Can you work these out from the model? Positions are in its coordinate system, mm. A direction names the side the tool comes from. Round coordinates to 2 decimals unless told otherwise and drop trailing zeros. Order: outer loops, then holes, each group sorted by start corner. A loop starts at its lowest first (then second) coordinate and runs counter-clockwise, first axis right, second up. Notation, with made-up numbers: M 25.5,56 L 78.5,56 A11 ccw 78.5,74 Z; hole C 51.25,87 d10. An arc over 180 degrees is marked long. Answer as a JSON object with one key per item and string values. Group by question number.
from build123d import *

# Parameters (mm, degrees)
CROQUIS1_W              = 38.1
CROQUIS1_H              = 700
SALIENTE_EXTRUIR1_DEPTH = 3.2
CROQUIS2_W              = 3.2
CROQUIS2_H              = 700
SALIENTE_EXTRUIR2_DEPTH = 34.9
CROQUIS5_R              = 3.175
CORTAR_EXTRUIR1_DEPTH   = 10
CROQUIS6_R              = 3.175
CORTAR_EXTRUIR2_DEPTH   = 10


with BuildPart() as part:
    # Croquis1 → Saliente-Extruir1 (new body)
    with BuildSketch(Plane.XY):
        with Locations((-19.05, 350)):
            Rectangle(CROQUIS1_W, CROQUIS1_H)
    extrude(amount=SALIENTE_EXTRUIR1_DEPTH)

    # Croquis2 → Saliente-Extruir2 (add)
    with BuildSketch(Plane.XY.offset(3.2)):
        with Locations((-36.5, 350)):
            Rectangle(CROQUIS2_W, CROQUIS2_H)
    extrude(amount=SALIENTE_EXTRUIR2_DEPTH)

    # Croquis5 → Cortar-Extruir1 (cut)
    with BuildSketch(Plane.XY.offset(3.2)):
        with Locations((-16.9, 673)):
            Circle(CROQUIS5_R)
        with Locations((-16.9, 657)):
            Circle(CROQUIS5_R)
        with Locations((-16.9, 208)):
            Circle(CROQUIS5_R)
        with Locations((-16.9, 192)):
            Circle(CROQUIS5_R)
    extrude(amount=-CORTAR_EXTRUIR1_DEPTH, mode=Mode.SUBTRACT)

    # Croquis6 → Cortar-Extruir2 (cut)
    with BuildSketch(Plane(origin=(-34.9, 0, 0), x_dir=(0, 0, -1), z_dir=(1, 0, 0))):
        with Locations((-21.2, 626)):
            Circle(CROQUIS6_R)
        with Locations((-21.2, 610)):
            Circle(CROQUIS6_R)
        with Locations((-21.2, 166)):
            Circle(CROQUIS6_R)
        with Locations((-21.2, 150)):
            Circle(CROQUIS6_R)
    extrude(amount=-CORTAR_EXTRUIR2_DEPTH, mode=Mode.SUBTRACT)


solid = part.part
Item 1: Suppose I cut it at B-B, the plane z = 12. Write out the boundary of the cut face in (x, y), and give its area (3 significant figures).
Item 2: I need wall thicknesses on line 1 (Y direction, x = -36.35, z = 21.2) (3 decimals); line 2 (Y direction, x = -16.9, z = 1.8) (3 decimals); line 3 (Z direction, x = -36, y = 626) (3 decimals). Which ranges of each line are inside material? Lowest first, please.
Item 3: I'm going to push flat-ended pins straight in: pin 1 Ø2 at (x, y) = (-21.5, 210) entering from +Z; pin 2 Ø10.5 at (y, z) = (211, 15) entering from +X. Where does each tip first touch, or does it pass through?
Item 4: Suppose I cut it at A-A, the plane y = 580.5. Write out the boundary of the cut face in (x, z).
Item 5: On a 3-axis mill with a long thin cutter (end or side, diameter ignored), from which of +Z, -Z, +X, -X, +Y, -Y can I reach the whole of each face in a straight line? I mean faces 1 (the face through (-36, 0, 10)), 2 (the face through (-18, 355, 3.2)). Say none if no direction works.
Computed:
{
 "1": {"outline": "M -38.1,0 L -34.9,0 L -34.9,700 L -38.1,700 Z", "area": "2,240 mm^2"},
 "2": {"line 1": "y = 0 to 146.825, 153.175 to 162.825, 169.175 to 606.825, 613.175 to 622.825, 629.175 to 700", "line 2": "y = 0 to 188.825, 195.175 to 204.825, 211.175 to 653.825, 660.175 to 669.825, 676.175 to 700", "line 3": "z = 0 to 18.025, 24.375 to 38.1"},
 "3": {"pin 1": "stops at z = 3.2", "pin 2": "stops at x = -34.9"},
 "4": {"outline": "M -38.1,0 L 0,0 L 0,3.2 L -34.9,3.2 L -34.9,38.1 L -38.1,38.1 Z"},
 "5": {"face 1": "+Z, -Z, +X, -X, -Y", "face 2": "+Z, +X, +Y, -Y"}
}
